```python
from build123d import *

# Parameters (mm, degrees)
F0_W     = 25.4
F0_H     = 19.05
F1_DEPTH = 50.8
F2_R     = 1.5875
F4_DEPTH = 6.35
F3_R     = 1.5875
F5_DEPTH = 6.35


with BuildPart() as f1:
    # F0 (on Right) → F1 (new body)
    with BuildSketch(Plane.YZ):
        with Locations((-12.7, 9.525)):
            Rectangle(F0_W, F0_H)
        with BuildLine():
            ThreePointArc((0, 0), (9.525, 9.525), (0, 19.05))
            Line((0, 19.05), (0, 0))
        make_face()
    extrude(amount=F1_DEPTH)

    # F2 (on face) → F4 (join)
    with BuildSketch(Plane.YZ.offset(50.8)):
        with Locations((0, 9.525)):
            Circle(F2_R)
    extrude(amount=F4_DEPTH)

    # F3 (on face) → F5 (join)
    with BuildSketch(Plane(origin=(0, 0, 0), x_dir=(0, -1, 0), z_dir=(-1, 0, 0))):
        with Locations((0, 9.525)):
            Circle(F3_R)
    extrude(amount=F5_DEPTH)


solid = f1.part
```
Verification items for the finished model (mm, model axes). A direction names the side the tool comes from. Round coordinates to 2 decimals unless told otherwise and drop trailing zeros. Write each loop counter-clockwise with the first axis right and the second up, starting at its lowest first coordinate (ties: lowest second). Pieces come first, ordered by that corner, then holes. Notation, with made-up numbers: (-14.5, -38) - (27.5, -38) arc R23 cw to (27.5, -15) - close; hole circle Ø10 at (4, -37.75). An arc over 180 degrees is marked (long way). Answer as a JSON object with one key per item and string values. Group by question number.
Q1. Section check A-A, the plane x = 15.5. Enter the section's corners in (y, z) (3 decimals).
Q2. Section check B-B, the plane y = -14.5. Enter the section's corners in (x, z).
Q3. Go/stop test with flat-tipped pins: pin 1 Ø4 at (x, z) = (32.5, 6.5) entering from +Y; pin 2 Ø10 at (y, z) = (-7, 8) entering from +X; pin 3 Ø6 at (y, z) = (-8.5, 6.5) entering from -X. Record where each tip stops, or that it passes through.
Q4. Thickness scan on line 1 (X direction, y = -5.5, z = 17.75); line 2 (Y direction, x = 17.5, z = 11.25); line 3 (Y direction, x = 34.5, z = 16.25). Record the ranges inside material, lowest first.
Q5. Tool access check on faces 1 (the cylindrical face through (25.044, 9.523, 9.316)), 2 (the cylindrical face through (53.931, -0.344, 7.975)), 3 (the cylindrical face through (-3.131, 0.344, 7.975)). Record the directions out of +Z, -Z, +X, -X, +Y, -Y that give a thin tool (end or side, any length) a straight path to the whole face; none if there is none.
Found:
{
 "1": {"outline": "(-25.4, 0) - (0, 0) arc R9.525 ccw to (0, 19.05) - (-25.4, 19.05) - close"},
 "2": {"outline": "(0, 0) - (50.8, 0) - (50.8, 19.05) - (0, 19.05) - close"},
 "3": {"pin 1": "stops at y = 9.47", "pin 2": "stops at x = 50.8", "pin 3": "stops at x = 0"},
 "4": {"line 1": "x = 0 to 50.8", "line 2": "y = -25.4 to 9.37", "line 3": "y = -25.4 to 6.75"},
 "5": {"face 1": "+X, -X, +Y", "face 2": "+X", "face 3": "-X"}
}
